Can you work these out from the drawing? Everything is in mm from the part's minimum corner. Give positions to 0.01 mm unless a question says otherwise; leave off trailing zeros. Write each loop counter-clockwise with the first axis right and the second up, starting at its lowest first coordinate (ties: lowest second). Pieces come first, ordered by that corner, then holes. Notation, with made-up numbers: (-24, 39) - (27, 39) arc R19 cw to (27, 73) - close; hole circle Ø6 at (13, -18.5). An arc over 180 degrees is marked (long way). Return JSON: item names as keys, results as strings. Group by question number.
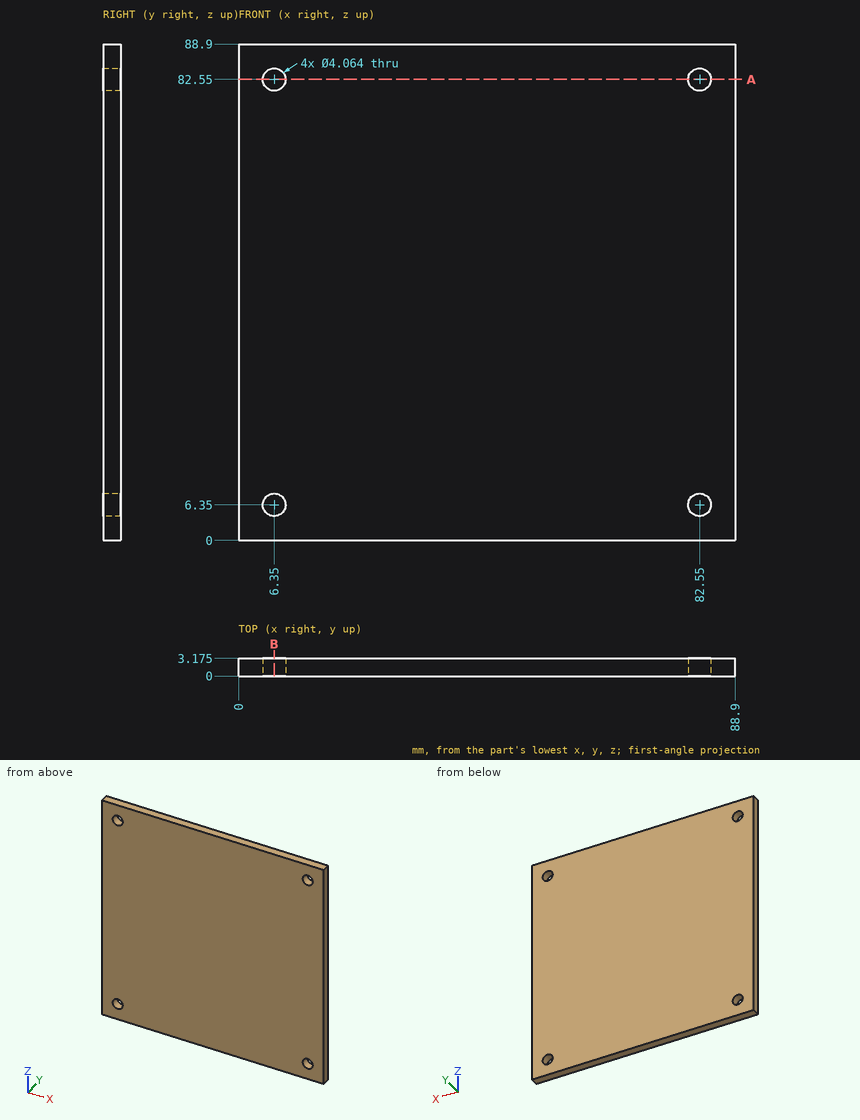
1) Imagine slicing it at B-B, the plane x = 6.35. Write out the boundary of the cut face in (y, z) (3 decimals), and give its area (3 significant figures).
2) Imagine slicing it at A-A, the plane z = 82.55. Write out the boundary of the cut face in (x, y) (3 decimals).
3) I need wall thicknesses on line 1 along X through (y, z) = (1.6, 6.35). Which ranges of the line are inside material? Lowest first, please.
4) Will these pins go through, and if not, where does the flat tip stop? pin 1 Ø6.5 at (x, z) = (82.55, 6.35) entering from -Y; pin 2 Ø3.5 at (x, z) = (82.55, 82.55) entering from +Y.
Resolved:
{
 "1": {"outline": "(0, 0) - (3.175, 0) - (3.175, 4.318) - (0, 4.318) - close; (0, 8.382) - (3.175, 8.382) - (3.175, 80.518) - (0, 80.518) - close; (0, 84.582) - (3.175, 84.582) - (3.175, 88.9) - (0, 88.9) - close", "area": "256 mm^2"},
 "2": {"outline": "(0, 0) - (4.318, 0) - (4.318, 3.175) - (0, 3.175) - close; (8.382, 0) - (80.518, 0) - (80.518, 3.175) - (8.382, 3.175) - close; (84.582, 0) - (88.9, 0) - (88.9, 3.175) - (84.582, 3.175) - close"},
 "3": {"line 1": "0 to 4.32, 8.38 to 80.52, 84.58 to 88.9"},
 "4": {"pin 1": "y = 0", "pin 2": "through"}
}
